Build history of the part. All positions in model axes, mm. A direction names the side the tool comes from. Give positions to 0.01 mm unless a question says otherwise; leave off trailing zeros. Order: outer loops, then holes, each group sorted by start corner. A loop starts at its lowest first (then second) coordinate and runs counter-clockwise, first axis right, second up. Notation, with made-up numbers: (51.5, 34.5) -> (73.5, 34.5) arc R32 ccw to (73.5, 72.5) -> close; hole circle Ø6 at (70.25, 6.25). An arc over 180 degrees is marked (long way). One line per item, written item: value. Start each with the question number.
(1) Probe line 1 (Y direction, x = -14.5, z = 0); line 2 (X direction, y = 4.5, z = -1). List the from-to ranges inside material, lowest first.
(2) Saw through at D-D on z = -5.75. Give the cut face in (x, y), plus the area to 3 significant figures.
(3) Saw through at C-C on x = -0.75. Give the cut face in (y, z), plus the area to 3 significant figures.
(4) Two-plate mould, pull along X, no slides. Class faces 1 (the flat face through (0, 25, 15)), 2 (the flat face through (0, 25, -13.3)), 3 (the flat face through (-15, 25, 0)): +X half, -X half, draft (parallel to the pull), parting line (faces both ways), or undercut.
(5) Which spindle directions (+Z, -Z, +X, -X, +Y, -Y) get a long thin tool onto all of the face, cutting with end or side? Do faces 4 (the flat face through (13.3, 25, 0)), 5 (the cylindrical face through (-14.4, 10.4, -0.4)), 6 (the cylindrical face through (14.41, 39.39, -0.89)). Say none if no direction does.
(6) Saw through at B-B on z = 0. Give the cut face in (x, y).
(7) Saw through at A-A on y = 46. Give the cut face in (x, z), plus the area to 3 significant figures.
(8) Pin check, flat tips, straight feed: pin 1 (6 mm diameter, centred on x = 8.5, z = -6.5, fed in from +Y); pin 2 (2 mm diameter, centred on y = 12, z = 0, fed in from -X); pin 3 (3 mm diameter, centred on y = 38, z = 0, fed in from +X). Stop position of each tip, or through.
```python
from build123d import *

# Parameters (mm, degrees)
SKETCH1_W           = 30
SKETCH1_H           = 30
BOSS_EXTRUDE1_DEPTH = 50
SHELL1_T            = -1.7
SKETCH2_R           = 1.65
CUT_EXTRUDE1_DEPTH  = 2
SKETCH3_R           = 1.65
CUT_EXTRUDE2_DEPTH  = 2
CHAMFER1_SIZE       = 0.5
CHAMFER2_SIZE       = 0.5


with BuildPart() as part:
    # Sketch1 → Boss-Extrude1 (new body)
    with BuildSketch(Plane(origin=(0, 0, 0), x_dir=(1, 0, 0), z_dir=(0, 1, 0))):
        Rectangle(SKETCH1_W, SKETCH1_H)
    extrude(amount=BOSS_EXTRUDE1_DEPTH)

    # Shell1
    shell1_openings = [part.faces().sort_by_distance(p)[0] for p in [
        (0, 50, 0),
        (0, 0, 0),
    ]]
    offset(amount=SHELL1_T, openings=shell1_openings, kind=Kind.INTERSECTION)

    # Sketch2 → Cut-Extrude1 (cut)
    with BuildSketch(Plane.ZY.offset(15)):
        with Locations((0, 12)):
            Circle(SKETCH2_R)
    extrude(amount=-CUT_EXTRUDE1_DEPTH, mode=Mode.SUBTRACT)

    # Sketch3 → Cut-Extrude2 (cut)
    with BuildSketch(Plane(origin=(15, 0, 0), x_dir=(0, 0, -1), z_dir=(1, 0, 0))):
        with Locations((0, 38)):
            Circle(SKETCH3_R)
    extrude(amount=-CUT_EXTRUDE2_DEPTH, mode=Mode.SUBTRACT)

    # Chamfer1
    chamfer1_edges = [part.edges().sort_by_distance(p)[0] for p in [
        (13.3, 38, 1.65),
    ]]
    chamfer(chamfer1_edges, length=CHAMFER1_SIZE)

    # Chamfer2
    chamfer2_edges = [part.edges().sort_by_distance(p)[0] for p in [
        (-13.3, 12, -1.65),
    ]]
    chamfer(chamfer2_edges, length=CHAMFER2_SIZE)


solid = part.part
```
Results below:
1. line 1: y = 0 to 10.35, 13.65 to 50
1. line 2: x = -15 to -13.3, 13.3 to 15
2. outline: (-15, 0) -> (-13.3, 0) -> (-13.3, 50) -> (-15, 50) -> close; (13.3, 0) -> (15, 0) -> (15, 50) -> (13.3, 50) -> close
2. area: 170 mm²
3. outline: (0, -15) -> (50, -15) -> (50, -13.3) -> (0, -13.3) -> close; (0, 13.3) -> (50, 13.3) -> (50, 15) -> (0, 15) -> close
3. area: 170 mm²
4. face 1: draft
4. face 2: undercut
4. face 3: -X half
5. face 4: +Y, -Y
5. face 5: -X
5. face 6: +X
6. outline: (-15, 0) -> (-13.3, 0) -> (-13.3, 9.85) -> (-13.8, 10.35) -> (-15, 10.35) -> close; (-15, 13.65) -> (-13.8, 13.65) -> (-13.3, 14.15) -> (-13.3, 50) -> (-15, 50) -> close; (13.3, 0) -> (15, 0) -> (15, 36.35) -> (13.8, 36.35) -> (13.3, 35.85) -> close; (13.3, 40.15) -> (13.8, 39.65) -> (15, 39.65) -> (15, 50) -> (13.3, 50) -> close
7. outline: (-15, -15) -> (15, -15) -> (15, 15) -> (-15, 15) -> close; hole (-13.3, -13.3) -> (13.3, -13.3) -> (13.3, 13.3) -> (-13.3, 13.3) -> close
7. area: 192 mm²
8. pin 1: passes through
8. pin 2: stops at x = 13.3
8. pin 3: stops at x = -13.3
